Can you work these out from the drawing? Everything is in mm from the part's minimum corner. A direction names the side the tool comes from. Coordinates: 2 decimals unless noted, no trailing zeros. Order: outer loops, then holes, each group sorted by start corner. A loop starts at its lowest first (then second) coordinate and runs counter-clockwise, first axis right, second up. Notation, with made-up numbers: (25.25, -8.75) -> (78.25, -8.75) arc R23 ccw to (78.25, 21.25) -> close; hole circle Ø11 at (-21, 32). An arc over 180 degrees is marked (long way). Answer in a Markdown table with one row per item.
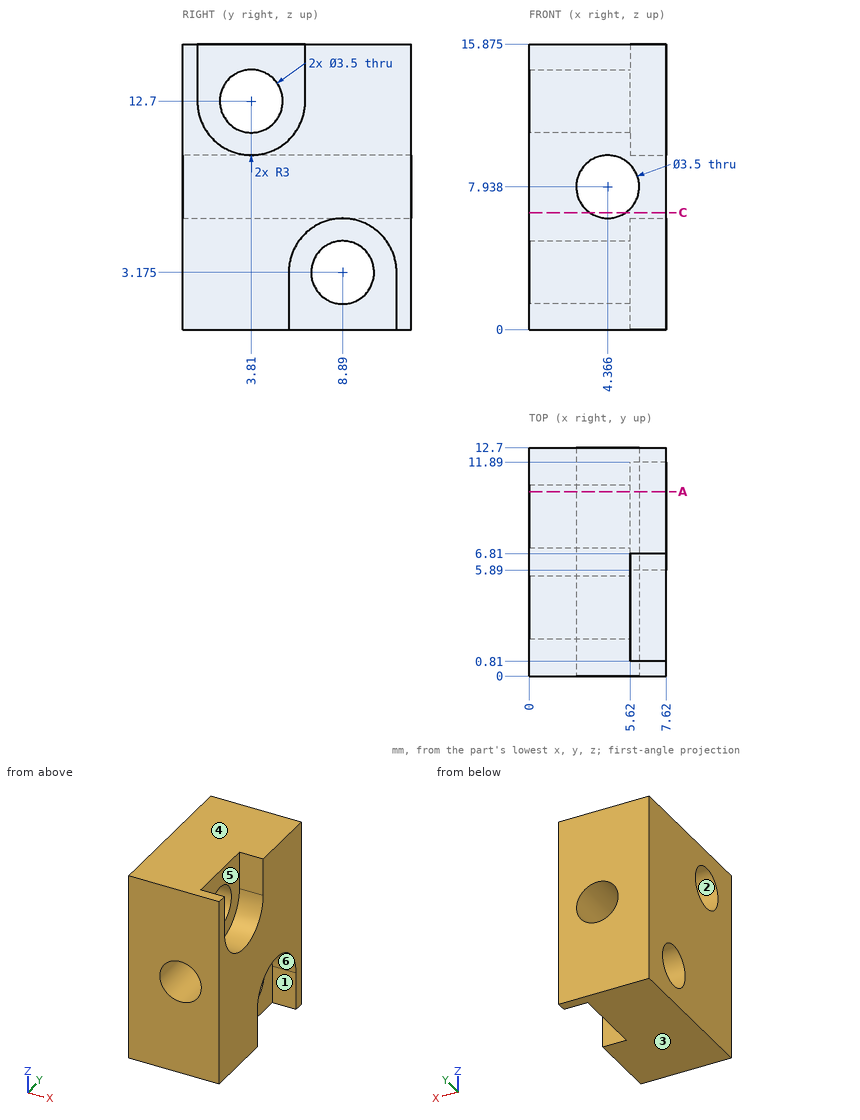
(1) We'd pull the mould along Z, two halves only. Please class the marked faces 1, 2 and 3: +Z half, -Z half, draft (parallel to the pull), parting line (faces both ways), or undercut.
Response values:
| item | result |
|---|---|
| face 1 | draft |
| face 2 | undercut |
| face 3 | -Z half |
(2) Suppose I cut it at A-A (y = 10.25). Count the separate pieces of the cut face and the enclosed holes in it.
Response values:
| item | result |
|---|---|
| separate pieces | 2 |
| enclosed holes | 1 |
(3) On a 3-axis mill with a long thin cutter (end or side, diameter ignored), from which of +Z, -Z, +X, -X, +Y, -Y can I reach the whole of each face in a straight line? I mean the marked faces 4, 5 and 6. Say none if no direction works.
Response values:
| item | result |
|---|---|
| face 4 | +Z, +X, -X, +Y, -Y |
| face 5 | +Z, +X |
| face 6 | -Z, +X |
(4) I need wall thicknesses on line 1 (Y direction, x = 7.5, z = 13.25); line 2 (Y direction, x = 3.55, z = 12.7); line 3 (Z direction, x = 3, y = 10.25) (1 decimal). Which ranges of each line are inside material? Lowest first, please. Write a range as [from, to].
Response values:
| item | result |
|---|---|
| line 1 | [0, 0.81], [6.81, 12.7] |
| line 2 | [0, 2.06], [5.56, 12.7] |
| line 3 | [0, 2.1], [4.3, 6.8], [9, 15.9] |
(5) Will this pin go through, and if not, where does the flat tip stop? pin 1 Ø3 at (y, z) = (3, 14) entering from +X.
Response values:
| item | result |
|---|---|
| pin 1 | x = 5.62 |
(6) Suppose I cut it at C-C (z = 6.5). Please give me the cut outline in (x, y) (1 decimal).
Response values:
| item | result |
|---|---|
| outline | (0, 0) -> (3.4, 0) -> (3.4, 12.7) -> (0, 12.7) -> close; (5.4, 0) -> (7.6, 0) -> (7.6, 12.7) -> (5.4, 12.7) -> close |
